Could you check a few things on this model? Use its own coordinates, in mm. Face numbers are marked on the shaded views. A direction names the side the tool comes from. Coordinates: 2 decimals unless noted, no trailing zeros. Loops run counter-clockwise (first coordinate to the right, second up) from the corner with the lowest first, then second, coordinate; pieces in that order, holes last. Notation, with made-up numbers: (51, 24.25) - (83, 24.25) arc R18 ccw to (83, 48.25) - close; hole circle Ø11 at (-22, -40). An arc over 180 degrees is marked (long way). One line per item, written item: value. Start each with the question number.
(1) If we section it at B-B on x = 27.7: Write out the boundary of the cut face in (y, z).
(2) If we section it at D-D on z = 1.75: Write out the boundary of the cut face in (x, y).
(3) If I drill on line 1 along Y through (x, z) = (-23.95, 10); line 2 along Y through (x, z) = (27.7, 2.85); line 3 along Z through (x, y) = (-24.4, 27.5), over which ranges is the centre line in solid material (lowest first)? Write a range as from..to.
(4) I'm going to push flat-ended pins straight in: P1, Ø6, axis at x = 20, y = 14, coming from the +Z side; P2, Ø5, axis at y = -12.5, z = 12, coming from the +X side. Where does each tip first touch, or does it pass through?
(5) If we section it at C-C on y = 27.5: Write out the boundary of the cut face in (x, z).
(6) On a 3-axis mill with a long thin cutter (end or side, diameter ignored), from which of +Z, -Z, +X, -X, +Y, -Y can I reach the whole of each face in a straight line? I mean the marked faces 1 and 2. Say none if no direction works.
(7) If we section it at A-A on z = 10: Write out the boundary of the cut face in (x, y), then the cut area to 3 significant figures.
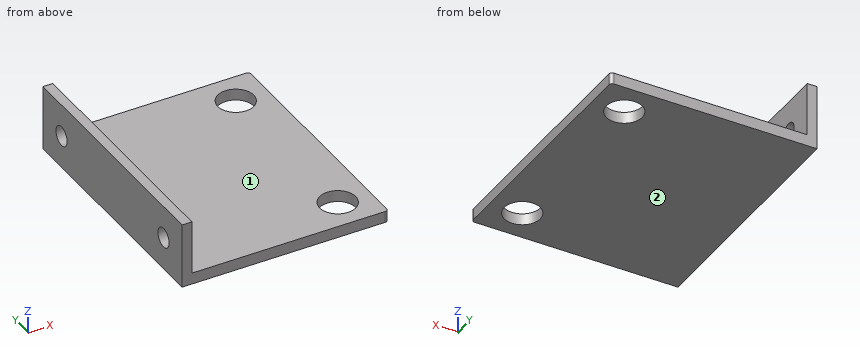
Autodesk Inventor part; units mm, degrees
ref_plane "Work Plane2" through (-30.7961, -197.5, 20) normal (0, 0, 1) x (1, 0, 0)
ref_plane "YZ Plane" through (0, 0, 0) normal (1, 0, 0) x (0, 1, 0)
ref_plane "XZ Plane" through (0, 0, 0) normal (0, 1, 0) x (-1, 0, 0)
ref_plane "Work Plane1" through (0, 0, 0) normal (0, 0, 1) x (1, 0, 0)
sketch "Sketch1" plane through (0, 0, 0) normal (0, 0, 1) x (1, 0, 0)
  line L0 (-36.5, 37.5) -> (36.5, 37.5)
  arc A0 (37.5, 36.5) -> (36.5, 37.5) centre (36.5, 36.5) ccw
  line L1 (37.5, 36.5) -> (37.5, -36.5)
  line L2 (36.5, -37.5) -> (-36.5, -37.5)
  arc A1 (36.5, -37.5) -> (37.5, -36.5) centre (36.5, -36.5) ccw
  line L3 (37.5, 37.5) -> (-25.4999, 37.5)
  line L4 (-25.4999, 37.5) -> (-25.4999, -37.5)
  line L5 (-25.4999, -37.5) -> (37.5, -37.5)
  line L6 (37.5, -37.5) -> (37.5, 37.5)
  circle A2 centre (27.7, 27.5) radius 5.5
  circle A3 centre (27.7, -27.5) radius 5.5
  point P0 (0, 0)
  point P1 (-25.4999, 37.5)
extrude "Extrusion1" add sketch "Sketch1" along normal blind 3.5 contours L0 A0 L1 A1 L2 L4
sketch "Sketch2" plane through (0, 0, 3.5) normal (0, 0, 1) x (1, 0, 0)
  line L0 (-25.4999, 37.5) -> (-25.4999, -37.5)
  line L1 (-25.4999, -37.5) -> (36.5, -37.5)
  line L2 (-25.4999, 37.5) -> (-22.4999, 37.5)
  line L3 (-22.4999, 37.5) -> (-22.4999, -37.5)
  line L4 (-22.4999, -37.5) -> (-25.4999, -37.5)
  line L5 (-25.4999, -37.5) -> (-25.4999, 37.5)
  point P0 (0, 0)
  dimension "d2" = 3
ref_plane "Work Plane2" through (-30.7961, -197.5, 20) normal (0, 0, 1) x (1, 0, 0)
extrude "Extrusion2" add sketch "Sketch2" along normal blind 16.5
sketch "Sketch3" plane through (-22.4999, -37.5, 3.5) normal (1, 0, 0) x (0, 0, -1)
  circle A0 centre (-6.5, 65) radius 3
  circle A1 centre (-6.5, 10) radius 3
  line L0 (-6.5, 10) -> (-6.5, 65)
  line L1 (0, 75) -> (-16.5, 75)
  line L2 (0, 0) -> (-16.5, 0)
  line L3 (-16.5, 0) -> (-16.5, 75)
  point P0 (3.5, 37.5)
  point P1 (-6.5, 37.5)
  dimension "d5" = 6
  dimension "d6" = 6
  dimension "d7" = 10
  dimension "d8" = 10
  dimension "d9" = 10
extrude "Extrusion3" cut sketch "Sketch3" against normal blind 16.5
properties part number "BackPistonSupport Top"
Values:
1. outline: (-37.5, 0) - (-33, 0) - (-33, 3.5) - (-37.5, 3.5) - close; (-22, 0) - (22, 0) - (22, 3.5) - (-22, 3.5) - close; (33, 0) - (37.5, 0) - (37.5, 3.5) - (33, 3.5) - close
2. outline: (-25.5, -37.5) - (36.5, -37.5) arc R1 ccw to (37.5, -36.5) - (37.5, 36.5) arc R1 ccw to (36.5, 37.5) - (-25.5, 37.5) - close; hole circle Ø11 at (27.7, -27.5); hole circle Ø11 at (27.7, 27.5)
3. line 1: y = -37.5..-30.5, -24.5..24.5, 30.5..37.5
3. line 2: y = -37.5..-33, -22..22, 33..37.5
3. line 3: z = 0..7, 13..20
4. P1: stops at z = 3.5
4. P2: stops at x = -22.5
5. outline: (-25.5, 0) - (22.2, 0) - (22.2, 3.5) - (-22.5, 3.5) - (-22.5, 7) - (-25.5, 7) - close; (-25.5, 13) - (-22.5, 13) - (-22.5, 20) - (-25.5, 20) - close; (33.2, 0) - (37.5, 0) - (37.5, 3.5) - (33.2, 3.5) - close
6. face 1: +Z, +X, +Y, -Y
6. face 2: -Z, +X, -X, +Y, -Y
7. outline: (-25.5, -37.5) - (-22.5, -37.5) - (-22.5, -30.5) - (-25.5, -30.5) - close; (-25.5, -24.5) - (-22.5, -24.5) - (-22.5, 24.5) - (-25.5, 24.5) - close; (-25.5, 30.5) - (-22.5, 30.5) - (-22.5, 37.5) - (-25.5, 37.5) - close
7. area: 189 mm2
